from build123d import *

# Parameters (mm, degrees)
F1_DEPTH = 4.7
F2_W     = 0.5
F2_H     = 0.25
F3_DEPTH = 2


with BuildPart() as f1:
    # F0 (on Right) → F1 (new body)
    with BuildSketch(Plane.YZ):
        with BuildLine():
            ThreePointArc((13.7373347581, 2.2654625069), (11.6220312193, 2.4917482212), (9.5067276805, 2.2654625069))
            ThreePointArc((9.5067276805, 2.2654625069), (11.6220312193, -1.1082517788), (13.7373347581, 2.2654625069))
        make_face()
    extrude(amount=F1_DEPTH)

    # F2 (on face) → F3 (join)
    with BuildSketch(Plane.YZ.offset(4.7)):
        with Locations((10.6020312193, 1.1167482212)):
            Rectangle(F2_W, F2_H)
        with Locations((11.6220312193, 1.1167482212)):
            Rectangle(F2_W, F2_H)
        with Locations((12.6420312193, 1.1167482212)):
            Rectangle(F2_W, F2_H)
    extrude(amount=F3_DEPTH)


solid = f1.part
Can you work these out from the model? Positions are in its coordinate system, mm. Round coordinates to 2 decimals unless told otherwise and drop trailing zeros. Order: outer loops, then holes, each group sorted by start corner. A loop starts at its lowest first (then second) coordinate and runs counter-clockwise, first axis right, second up. Notation, with made-up numbers: (77, 18) - (108, 18) arc R15 cw to (108, 43) - close; hole circle Ø5 at (57.5, -9.75). An arc over 180 degrees is marked (long way). Answer in a Markdown table with one row per item.
(1) For P1, Ø1.5, axis at x = 2.5, z = 1, coming from the +Y side, with a flat end and sliding along its axis, tell me the tip position at first contact or that it passes through.
From the geometry:
| item | result |
|---|---|
| P1 | stops at y = 13.97 |
(2) If we mould it in two halves opening along X, with no side actions, what happens to faces 1 (the face through (2.317, 11.556, -1.107)), 2 (the face through (0, 12, 1))? For each: released by +X, released by -X, zero draft, split by the parting line, or undercut.
From the geometry:
| item | result |
|---|---|
| face 1 | zero draft |
| face 2 | released by -X |
(3) Suppose I cut it at A-A, the plane x = 5. Please give me the cut outline in (y, z), plus the area to 3 significant figures.
From the geometry:
| item | result |
|---|---|
| outline | (10.35, 0.99) - (10.85, 0.99) - (10.85, 1.24) - (10.35, 1.24) - close; (11.37, 0.99) - (11.87, 0.99) - (11.87, 1.24) - (11.37, 1.24) - close; (12.39, 0.99) - (12.89, 0.99) - (12.89, 1.24) - (12.39, 1.24) - close |
| area | 0.375 mm2 |
(4) Please list where these lines run through material, in increasing order: L1, parallel to Y at x = 6.5, z = 1.1; L2, parallel to X at y = 12.15, z = 0.4; L3, parallel to Z at x = 5.5, y = 12.75. Write a range as from..to.
From the geometry:
| item | result |
|---|---|
| L1 | y = 10.35..10.85, 11.37..11.87, 12.39..12.89 |
| L2 | x = 0..4.7 |
| L3 | z = 0.99..1.24 |
(5) Suppose I cut it at C-C, the plane z = 2.05. Please give me the cut outline in (x, y).
From the geometry:
| item | result |
|---|---|
| outline | (0, 9.42) - (4.7, 9.42) - (4.7, 13.83) - (0, 13.83) - close |
(6) Suppose I cut it at D-D, the plane x = 2.75. Please give me the cut outline in (y, z), plus the area to 3 significant figures.
From the geometry:
| item | result |
|---|---|
| outline | (9.51, 2.27) arc R2.35 ccw (long way) to (13.74, 2.27) arc R10 ccw to start |
| area | 14.0 mm2 |
(7) Suppose I cut it at B-B, the plane y = 10.55. Please give me the cut outline in (x, z), plus the area to 3 significant figures.
From the geometry:
| item | result |
|---|---|
| outline | (0, -0.85) - (4.7, -0.85) - (4.7, 0.99) - (6.7, 0.99) - (6.7, 1.24) - (4.7, 1.24) - (4.7, 2.43) - (0, 2.43) - close |
| area | 15.9 mm2 |
